For this review, take the finished solid that the model builds, in its own axes (mm). A direction names the side the tool comes from. Round coordinates to 2 decimals unless told otherwise and drop trailing zeros. Write each loop counter-clockwise with the first axis right and the second up, starting at its lowest first coordinate (ties: lowest second). Pieces come first, ordered by that corner, then holes. Notation, with made-up numbers: (37, 52.5) - (69, 52.5) arc R26 ccw to (69, 77.5) - close; hole circle Ø3 at (-3.5, 53.25). An arc over 180 degrees is marked (long way). Answer in a Markdown table with one row per item. Add a question column.
from build123d import *

# Parameters (mm, degrees)
CHAMFER_2_SIZE = 2


with BuildPart() as part:
    # Эскиз1 → Повернуть1 (revolve)
    with BuildSketch(Plane(origin=(0, 0, 0), x_dir=(0, 0, -1), z_dir=(1, 0, 0)), mode=Mode.PRIVATE) as revolve_1_sk:
        Polygon((-84.15, 50), (-103, 50), (-103, 68), (-18, 68), (-18, 72.5), (0, 72.5), (0, 60), (-9.85, 60), (-9.85, 62), (-14, 62), (-14, 60), (-63, 60), (-63, 50), (-66, 50), (-66, 41), (-71, 41), (-71, 50), (-81, 50), (-81, 51.75), (-84.15, 51.75), align=None)
    revolve(revolve_1_sk.sketch.rotate(Axis((0, 0, 0), (0, 0, 1)), 90), axis=Axis((0, 0, 0), (0, 0, 1)))

    # Фаска2
    chamfer_2_edges = [part.edges().sort_by_distance(p)[0] for p in [
        (50, 0, 103),
        (60, 0, 0),
        (72.5, 0, 0),
        (68, 0, 103),
    ]]
    chamfer(chamfer_2_edges, length=CHAMFER_2_SIZE)


solid = part.part
Q1. To check wall thickness, follow probe 1 along Y at (x, z) = (-2, 20); probe 2 along Z at (x, y) = (-46.5, -17); probe 3 along X at (y, z) = (1, 79). State the ranges of each line that lie inside material, in increasing order.
Q2. Add section B-B on z = 89. State the section outline as (x, y) points.
Q3. Insertion check: pin 1 Ø12 at (x, y) = (-24, 42.5) entering from -Z; pin 2 Ø3 at (y, z) = (9.5, 62.5) entering from -X; pin 3 Ø10 at (x, z) = (-45, 17.5) entering from +Y. Each pin has a flat end and moves straight along its axis. Give the tip position at first contact, or say it passes through.
Q4. Add section A-A on z = 55.5. State the section outline as (x, y) points, then the cut area to 3 significant figures.
Q5. Draft analysis for pull direction Y (two halves, no side actions). For faces 5 (the face through (-47.69, -15.02, 64.52)), 6 (the face through (21, -65, 18)), 7 (the face through (-47.69, -15.02, 92.69)), 8 (the face through (8.85, -67.42, 58.92)), state which applies: released by +Y, released by -Y, zero draft, split by the parting line, or undercut.
Q6. Tool access review of faces 1 (the face through (-47.69, -15.02, 76.07)), 2 (the face through (23, -45, 63)), 3 (the face through (32, -51, 14)), 4 (the face through (0.3, 62.3, 0)): name each direction out of +Z, -Z, +X, -X, +Y, -Y from which nothing blocks a thin tool from reaching the whole face with its end or side.
Answer sheet:
| question | item | result |
|---|---|---|
| 1 | probe 1 | y = -67.97 to -59.97, 59.97 to 67.97 |
| 1 | probe 2 | z = 66 to 71 |
| 1 | probe 3 | x = -67.99 to -49.99, 49.99 to 67.99 |
| 2 | outline | circle Ø136 at (0, 0); hole circle Ø100 at (0, 0) |
| 3 | pin 1 | stops at z = 63 |
| 3 | pin 2 | stops at x = -67.53 |
| 3 | pin 3 | stops at y = 60.47 |
| 4 | outline | circle Ø136 at (0, 0); hole circle Ø120 at (0, 0) |
| 4 | area | 3,220 mm² |
| 5 | face 5 | undercut |
| 5 | face 6 | zero draft |
| 5 | face 7 | undercut |
| 5 | face 8 | split by the parting line |
| 6 | face 1 | +Z |
| 6 | face 2 | -Z |
| 6 | face 3 | none |
| 6 | face 4 | -Z, +X, -X, +Y, -Y |
